from build123d import *

# Parameters (mm, degrees)
F0_W          = 106
F0_H          = 100
F1_DEPTH      = 4
F2_W          = 82
F2_H          = 94
F2_W_2        = 78
F2_H_2        = 90
F5_DEPTH      = 2
F6_DEPTH      = 25
F4_R          = 5
F4_R_2        = 2
F7_DEPTH      = 4
F8_W          = 6
F8_H          = 6
F9_DEPTH      = 5
F10_R         = 1.5
F11_DEPTH     = 5
F12_W         = 6
F12_H         = 6
F13_DEPTH     = 5
F14_R         = 1.5
F15_DEPTH     = 5
F16_R         = 5
F17_T1_DEPTH  = 90
F17_T3_DEPTH  = 96
F17_T6_ANGLE  = 90
F17_T8_ANGLE  = 90
F17_T10_ANGLE = 90
F17_T12_ANGLE = 90


# Not quite as in the source:
# - a fillet or chamfer that OpenCascade refuses, or shapes differently, is made with other operations: its cross-section is extruded or revolved along the edge and cut away or added


with BuildPart() as f1:
    # F0 (on Top) → F1 (new body)
    with BuildSketch(Plane.XY):
        with Locations((-29.9393483698, 26.8405017372)):
            Rectangle(F0_W, F0_H)
    extrude(amount=F1_DEPTH)

    # F2 (on face) → F5 (join)
    with BuildSketch(Plane.XY.offset(4)):
        with Locations((-29.9393483698, 26.8405017372)):
            Rectangle(F2_W, F2_H)
        with Locations((-29.9393483698, 26.8405017372)):
            Rectangle(F2_W_2, F2_H_2, mode=Mode.SUBTRACT)
    extrude(amount=F5_DEPTH)

    # F3 (on face) → F6 (cut)
    with BuildSketch(Plane.XY.offset(4)):
        with BuildLine():
            ThreePointArc((-77.9393483698, 49.7999965698), (-76.5251348075, 50.3857830074), (-75.9393483698, 51.7999965698))
            ThreePointArc((-75.9393483698, 51.7999965698), (-76.5251348075, 53.2142101321), (-77.9393483698, 53.7999965698))
            Line((-77.9393483698, 53.7999965698), (-77.9393483698, 51.7999965698))
            Line((-77.9393483698, 51.7999965698), (-77.9393483698, 49.7999965698))
        make_face()
        with BuildLine():
            ThreePointArc((-75.9393483698, 1.7999965698), (-76.5251348075, 3.2142101321), (-77.9393483698, 3.7999965698))
            Line((-77.9393483698, 3.7999965698), (-77.9393483698, 1.7999965698))
            Line((-77.9393483698, 1.7999965698), (-77.9393483698, -0.2000034302))
            ThreePointArc((-77.9393483698, -0.2000034302), (-76.5251348075, 0.3857830074), (-75.9393483698, 1.7999965698))
        make_face()
        with BuildLine():
            Line((-77.9393483698, 1.7999965698), (-77.9393483698, 3.7999965698))
            ThreePointArc((-77.9393483698, 3.7999965698), (-79.9393483698, 1.7999965698), (-77.9393483698, -0.2000034302))
            Line((-77.9393483698, -0.2000034302), (-77.9393483698, 1.7999965698))
        make_face()
        with BuildLine():
            ThreePointArc((-75.9393483698, 26.7999965698), (-76.5251348075, 28.2142101321), (-77.9393483698, 28.7999965698))
            Line((-77.9393483698, 28.7999965698), (-77.9393483698, 26.7999965698))
            Line((-77.9393483698, 26.7999965698), (-77.9393483698, 24.7999965698))
            ThreePointArc((-77.9393483698, 24.7999965698), (-76.5251348075, 25.3857830074), (-75.9393483698, 26.7999965698))
        make_face()
        with BuildLine():
            Line((-77.9393483698, 26.7999965698), (-77.9393483698, 28.7999965698))
            ThreePointArc((-77.9393483698, 28.7999965698), (-79.9393483698, 26.7999965698), (-77.9393483698, 24.7999965698))
            Line((-77.9393483698, 24.7999965698), (-77.9393483698, 26.7999965698))
        make_face()
        with BuildLine():
            Line((-77.9393483698, 51.7999965698), (-77.9393483698, 53.7999965698))
            ThreePointArc((-77.9393483698, 53.7999965698), (-79.9393483698, 51.7999965698), (-77.9393483698, 49.7999965698))
            Line((-77.9393483698, 49.7999965698), (-77.9393483698, 51.7999965698))
        make_face()
        with BuildLine():
            ThreePointArc((18.0606516302, 49.7999965698), (19.4748651925, 50.3857830074), (20.0606516302, 51.7999965698))
            ThreePointArc((20.0606516302, 51.7999965698), (19.4748651925, 53.2142101321), (18.0606516302, 53.7999965698))
            Line((18.0606516302, 53.7999965698), (18.0606516302, 51.7999965698))
            Line((18.0606516302, 51.7999965698), (18.0606516302, 49.7999965698))
        make_face()
        with BuildLine():
            ThreePointArc((20.0606516302, 1.7999965698), (19.4748651925, 3.2142101321), (18.0606516302, 3.7999965698))
            ThreePointArc((18.0606516302, 3.7999965698), (16.6464380678, 0.3857830074), (20.0606516302, 1.7999965698))
        make_face()
        with BuildLine():
            ThreePointArc((20.0606516302, 26.7999965698), (19.4748651925, 28.2142101321), (18.0606516302, 28.7999965698))
            Line((18.0606516302, 28.7999965698), (18.0606516302, 26.7999965698))
            Line((18.0606516302, 26.7999965698), (18.0606516302, 24.7999965698))
            ThreePointArc((18.0606516302, 24.7999965698), (19.4748651925, 25.3857830074), (20.0606516302, 26.7999965698))
        make_face()
        with BuildLine():
            Line((18.0606516302, 26.7999965698), (18.0606516302, 28.7999965698))
            ThreePointArc((18.0606516302, 28.7999965698), (16.0606516302, 26.7999965698), (18.0606516302, 24.7999965698))
            Line((18.0606516302, 24.7999965698), (18.0606516302, 26.7999965698))
        make_face()
        with BuildLine():
            Line((18.0606516302, 51.7999965698), (18.0606516302, 53.7999965698))
            ThreePointArc((18.0606516302, 53.7999965698), (16.0606516302, 51.7999965698), (18.0606516302, 49.7999965698))
            Line((18.0606516302, 49.7999965698), (18.0606516302, 51.7999965698))
        make_face()
    extrude(amount=-F6_DEPTH, mode=Mode.SUBTRACT)

    # F4 (on face) → F7 (join)
    with BuildSketch(Plane.XY.offset(4)):
        with Locations((-42.9393483698, 67.8405017372)):
            Circle(F4_R)
        with Locations((-42.9393483698, 67.8405017372)):
            Circle(F4_R_2, mode=Mode.SUBTRACT)
        with Locations((-29.9393483698, 67.8405017372)):
            Circle(F4_R)
        with Locations((-29.9393483698, 67.8405017372)):
            Circle(F4_R_2, mode=Mode.SUBTRACT)
        with Locations((-42.9393483698, -14.1594982628)):
            Circle(F4_R)
        with Locations((-42.9393483698, -14.1594982628)):
            Circle(F4_R_2, mode=Mode.SUBTRACT)
        with Locations((-29.9393483698, -14.1594982628)):
            Circle(F4_R)
        with Locations((-29.9393483698, -14.1594982628)):
            Circle(F4_R_2, mode=Mode.SUBTRACT)
    extrude(amount=F7_DEPTH)

    # F8 (on face) → F9 (join)
    with BuildSketch(Plane.XY.offset(4)):
        with Locations((-67.9393483698, 70.8405017372)):
            Rectangle(F8_W, F8_H)
        with Locations((-67.9393483698, -17.1594982628)):
            Rectangle(F8_W, F8_H)
    extrude(amount=F9_DEPTH)

    # F10 (on face) → F11 (cut)
    with BuildSketch(Plane(origin=(-70.9393483698, 0, 0), x_dir=(0, -1, 0), z_dir=(-1, 0, 0))):
        with Locations((-70.8405017372, 7)):
            Circle(F10_R)
        with Locations((17.1594982628, 7)):
            Circle(F10_R)
    extrude(amount=-F11_DEPTH, mode=Mode.SUBTRACT)

    # F12 (on face) → F13 (join)
    with BuildSketch(Plane.XY.offset(4)):
        with Locations((8.0606516302, 26.8405017372)):
            Rectangle(F12_W, F12_H)
    extrude(amount=F13_DEPTH)

    # F14 (on face) → F15 (cut)
    with BuildSketch(Plane.YZ.offset(11.0606516302)):
        with Locations((26.8405017372, 7)):
            Circle(F14_R)
    extrude(amount=-F15_DEPTH, mode=Mode.SUBTRACT)

    # F16
    f16_edges = [f1.edges().sort_by_distance(p)[0] for p in [
        (-82.939348, 76.840502, 2),
        (23.060652, 76.840502, 2),
        (23.060652, -23.159498, 2),
        (-82.939348, -23.159498, 2),
    ]]
    fillet(f16_edges, radius=F16_R)

    # F17: fillet of radius 4 on 8 edges, made by hand

    # F17_s2 → F17_t1 (cut)
    with BuildSketch(Plane.XZ.offset(-71.8405017372)):
        with BuildLine():
            ThreePointArc((23.0606516302, 4), (21.8890787549, 1.1715728753), (19.0606516302, 0))
            Line((19.0606516302, 0), (23.0606516302, 0))
            Line((23.0606516302, 0), (23.0606516302, 4))
        make_face()
        with BuildLine():
            ThreePointArc((-78.9393483698, 0), (-81.7677754946, 1.1715728753), (-82.9393483698, 4))
            Line((-82.9393483698, 4), (-82.9393483698, 0))
            Line((-82.9393483698, 0), (-78.9393483698, 0))
        make_face()
    extrude(amount=F17_T1_DEPTH, mode=Mode.SUBTRACT)

    # F17_s4 → F17_t3 (cut)
    with BuildSketch(Plane.YZ.offset(-77.9393483698)):
        with BuildLine():
            ThreePointArc((-19.1594982628, 0), (-21.9879253875, 1.1715728753), (-23.1594982628, 4))
            Line((-23.1594982628, 4), (-23.1594982628, 0))
            Line((-23.1594982628, 0), (-19.1594982628, 0))
        make_face()
        with BuildLine():
            ThreePointArc((72.8405017372, 0), (75.668928862, 1.1715728753), (76.8405017372, 4))
            Line((76.8405017372, 4), (76.8405017372, 0))
            Line((76.8405017372, 0), (72.8405017372, 0))
        make_face()
    extrude(amount=F17_T3_DEPTH, mode=Mode.SUBTRACT)

    # F17_s5 → F17_t6 (revolve, cut)
    with BuildSketch(Plane.XZ.offset(18.1594982628)):
        with BuildLine():
            ThreePointArc((19.0606516302, 0), (21.8890787549, 1.1715728753), (23.0606516302, 4))
            Line((23.0606516302, 4), (23.0606516302, 0))
            Line((23.0606516302, 0), (19.0606516302, 0))
        make_face()
    revolve(axis=Axis((18.0606516302, -18.1594982628, 0), (0, 0, -1)), revolution_arc=F17_T6_ANGLE, mode=Mode.SUBTRACT)

    # F17_s7 → F17_t8 (revolve, cut)
    with BuildSketch(Plane.XZ.offset(-71.8405017372)):
        with BuildLine():
            ThreePointArc((19.0606516302, 0), (21.8890787549, 1.1715728753), (23.0606516302, 4))
            Line((23.0606516302, 4), (23.0606516302, 0))
            Line((23.0606516302, 0), (19.0606516302, 0))
        make_face()
    revolve(axis=Axis((18.0606516302, 71.8405017372, 0), (0, 0, 1)), revolution_arc=F17_T8_ANGLE, mode=Mode.SUBTRACT)

    # F17_s9 → F17_t10 (revolve, cut)
    with BuildSketch(Plane.YZ.offset(-77.9393483698)):
        with BuildLine():
            ThreePointArc((-19.1594982628, 0), (-21.9879253875, 1.1715728753), (-23.1594982628, 4))
            Line((-23.1594982628, 4), (-23.1594982628, 0))
            Line((-23.1594982628, 0), (-19.1594982628, 0))
        make_face()
    revolve(axis=Axis((-77.9393483698, -18.1594982628, 0), (0, 0, -1)), revolution_arc=F17_T10_ANGLE, mode=Mode.SUBTRACT)

    # F17_s11 → F17_t12 (revolve, cut)
    with BuildSketch(Plane.YZ.offset(-77.9393483698)):
        with BuildLine():
            ThreePointArc((72.8405017372, 0), (75.668928862, 1.1715728753), (76.8405017372, 4))
            Line((76.8405017372, 4), (76.8405017372, 0))
            Line((76.8405017372, 0), (72.8405017372, 0))
        make_face()
    revolve(axis=Axis((-77.9393483698, 71.8405017372, 0), (0, 0, 1)), revolution_arc=F17_T12_ANGLE, mode=Mode.SUBTRACT)


solid = f1.part
Geometry: final body of the model. Coordinates: model frame, mm. A direction names the side the tool comes from. Coordinates: 2 decimals unless noted, no trailing zeros. Loops run counter-clockwise (first coordinate to the right, second up) from the corner with the lowest first, then second, coordinate; pieces in that order, holes last. Notation, with made-up numbers: (69.5, 55.25) - (115.5, 55.25) arc R21 cw to (115.5, 79.25) - close; hole circle Ø6 at (55.5, 18). An arc over 180 degrees is marked (long way). One line per question, with ' | ' between items. Start each with the question number.
(1) First-contact query: pin 1 (3 mm diameter, centred on x = -22.5, y = 0, fed in from +Z); pin 2 (1.5 mm diameter, centred on y = 5, z = 6.5, fed in from +X); pin 3 (1.5 mm diameter, centred on x = -69.5, z = 7, fed in from +Y); pin 4 (5 mm diameter, centred on x = -45.5, z = 5, fed in from -Y). Flat tips, straight axial feed; report the tip coordinate or a pass-through.
(2) Ray query, L1, parallel to Y at x = -1, z = 4.75; L2, parallel to X at y = 6, z = 5; L3, parallel to Z at x = -18, y = -5.5. Return the intervals inside material, ascending. Write a range as from..to.
(3) Reachability of faces 5 (the flat face through (-68, 71, 9)), 6 (the cylindrical face through (8.596, 26.515, 5.536)), 7 (the cylindrical face through (-68.474, -18.545, 6.425)), 8 (the flat face through (11.061, 26, 5)), 9 (the flat face through (-67, -14.159, 6)) from +Z, -Z, +X, -X, +Y, -Y: full face, straight path, thin tool, end or side. Return the list, or none.
(4) Cut plane B-B on x = -8.5. Output: boundary loops of the cut face in (y, z), and give its area (3 significant figures).
(5) Cut plane C-C on z = 2. Count the separate pieces of the cut face and the enclosed holes in it, and give its area (3 significant figures).
(6) Cut plane A-A on y = 58. Output: boundary loops of the cut face in (x, z).
(7) Draft query along Y for faces 1 (the flat face through (-31, -20.159, 5)), 2 (the cylindrical face through (-28.03, 68.44, 5.97)), 3 (the cylindrical face through (21.92, 27.47, 1.2)), 4 (the cylindrical face through (-30.611, 75.638, 1.141)). Return one class per face: +Y half, -Y half, draft (parallel to the pull), parting line (faces both ways), or undercut.
Here are the results:
1) pin 1: z = 4 | pin 2: x = 11.06 | pin 3: y = 73.84 | pin 4: y = -23.16
2) L1: -20.16..-18.16, 71.84..73.84 | L2: -70.94..-68.94, 9.06..11.06 | L3: 0..4
3) face 5: +Z, +X, -X, +Y, -Y | face 6: +X | face 7: -X | face 8: +Z, +X, +Y, -Y | face 9: +Z
4) outline: (-23.16, 4) arc R4 ccw to (-19.16, 0) - (72.84, 0) arc R4 ccw to (76.84, 4) - (73.84, 4) - (73.84, 6) - (71.84, 6) - (71.84, 4) - (-18.16, 4) - (-18.16, 6) - (-20.16, 6) - (-20.16, 4) - close | area: 401 mm²
5) separate pieces: 1 | enclosed holes: 6 | area: 10,300 mm²
6) outline: (-82.94, 4) arc R4 ccw to (-78.94, 0) - (19.06, 0) arc R4 ccw to (23.06, 4) - (11.06, 4) - (11.06, 6) - (9.06, 6) - (9.06, 4) - (-68.94, 4) - (-68.94, 6) - (-70.94, 6) - (-70.94, 4) - close
7) face 1: -Y half | face 2: undercut | face 3: draft | face 4: +Y half
